Autodesk Inventor part; units mm, degrees
ref_plane "YZ Plane" through (0, 0, 0) normal (1, 0, 0) x (0, 1, 0)
ref_plane "XZ Plane" through (0, 0, 0) normal (0, 1, 0) x (-1, 0, 0)
ref_plane "XY Plane" through (0, 0, 0) normal (0, 0, 1) x (1, 0, 0)
sketch "Sketch1" plane through (0, 0, 0) normal (0, 1, 0) x (-1, 0, 0)
  circle A0 centre (0, 0) radius 55
  dimension "d4" = 110
sketch "Sketch2" plane through (0, 0, 0) normal (0, 1, 0) x (-1, 0, 0)
  circle A0 centre (0, 0) radius 40 construction
  circle A1 centre (0, 0) radius 47.5 construction
  circle A2 centre (0, 47.5) radius 4.5
  circle A3 centre (0, 47.5) radius 6.5
  dimension "d11" = 95
  dimension "d10" = 80
  dimension "d12" = 9
  dimension "d13" = 13
extrude "Extrusion1" add sketch "Sketch1" against normal blind 7
extrude "Extrusion2" add sketch "Sketch2" along normal blind 10
pattern_circular "Circular Pattern1" count 4 over 360 about axis through (0, -10, 0) along (0, 1, 0) of "Extrusion2"
sketch "Sketch3" plane through (0, -7, 0) normal (0, -1, 0) x (1, 0, 0)
  circle A0 centre (0, 0) radius 55
  circle A1 centre (0, 0) radius 55
  circle A2 centre (0, 0) radius 58
  dimension "d21" = 116
extrude "Extrusion3" add sketch "Sketch3" against normal blind 30
sketch "Sketch4" plane through (0, 0, 0) normal (0, 1, 0) x (1, 0, 0)
  circle A0 centre (0, 0) radius 12.5
  dimension "d24" = 25
extrude "Extrusion4" cut sketch "Sketch4" against normal blind 30
properties part number "BaseHumedadDireccion"
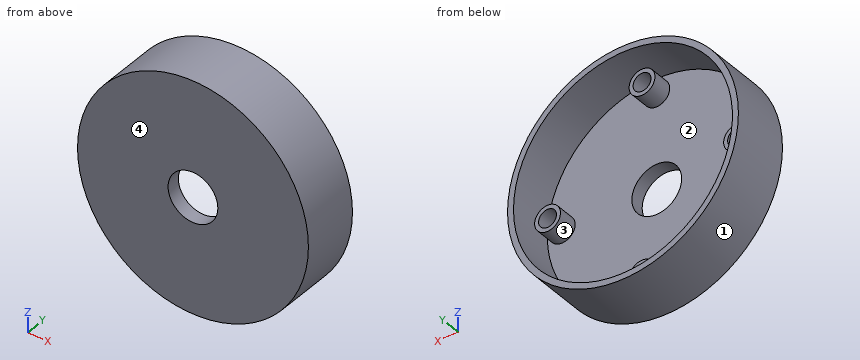
The listing builds one solid part. Answer for the finished solid, in the listing's coordinates (mm). Face numbers are marked on the shaded views. Give positions to 0.01 mm unless a question says otherwise; leave off trailing zeros. Order: outer loops, then holes, each group sorted by start corner. A loop starts at its lowest first (then second) coordinate and runs counter-clockwise, first axis right, second up. Notation, with made-up numbers: (77, -6) - (126, -6) arc R26 ccw to (126, 29) - close; hole circle Ø9 at (44.25, 46). An arc over 180 degrees is marked (long way). One line per item, written item: value. Start each with the question number.
1) A cutting plane is placed at A-A on z = 0. Give the vertices of the cut face in (x, y).
2) A cutting plane is placed at D-D on z = 35. Give the vertices of the cut face in (x, y).
3) Given pin 1 Ø20 at (x, z) = (0, 0) entering from +Y; pin 2 Ø4 at (x, z) = (-3, -46.5) entering from +Y; pin 3 Ø4 at (y, z) = (3, -5.5) entering from +X; pin 4 Ø1.5 at (x, y) = (-22.5, 2.5) entering from -Z, each flat-ended and moving along its own axis, determine where each tip first touches the part or whether it passes through.
4) A cutting plane is placed at B-B on x = -8. Give the vertices of the cut face in (y, z).
5) Find the intervals of material crossed by L1, parallel to Z at x = -47.5, y = 4.25; L2, parallel to Z at x = 0, y = -1.5; L3, parallel to X at y = 9, z = -50, in increasing order.
6) A cutting plane is placed at C-C on y = 11.75. Give the vertices of the cut face in (x, z).
7) The mould has two halves that part along X. Classify the marked faces 1, 2, 3 and 4: released by +X, released by -X, zero draft, split by the parting line, or undercut.
Answer sheet:
1. outline: (-58, -7) - (-12.5, -7) - (-12.5, 0) - (-41, 0) - (-41, 10) - (-43, 10) - (-43, 0) - (-52, 0) - (-52, 10) - (-54, 10) - (-54, 0) - (-55, 0) - (-55, 23) - (-58, 23) - close; (12.5, -7) - (58, -7) - (58, 23) - (55, 23) - (55, 0) - (54, 0) - (54, 10) - (52, 10) - (52, 0) - (43, 0) - (43, 10) - (41, 10) - (41, 0) - (12.5, 0) - close
2. outline: (-46.25, -7) - (46.25, -7) - (46.25, 23) - (42.43, 23) - (42.43, 0) - (-42.43, 0) - (-42.43, 23) - (-46.25, 23) - close
3. pin 1: passes through
3. pin 2: stops at y = 10
3. pin 3: stops at x = 57.89
3. pin 4: stops at z = -53.77
4. outline: (-7, -57.45) - (23, -57.45) - (23, -54.42) - (0, -54.42) - (0, -9.6) - (-7, -9.6) - close; (-7, 9.6) - (0, 9.6) - (0, 54.42) - (23, 54.42) - (23, 57.45) - (-7, 57.45) - close
5. L1: z = -33.28 to -27.73, -6.5 to -4.5, 4.5 to 6.5, 27.73 to 33.28
5. L2: z = -58 to -12.5, 12.5 to 58
5. L3: x = -29.39 to -22.91, -6 to -3.74, 3.74 to 6, 22.91 to 29.39
6. outline: circle Ø116 at (0, 0); hole circle Ø110 at (0, 0)
7. face 1: split by the parting line
7. face 2: undercut
7. face 3: undercut
7. face 4: zero draft
